Autodesk Inventor part; units mm, degrees
ref_plane "YZ Plane" through (0, 0, 0) normal (1, 0, 0) x (0, 1, 0)
ref_plane "XZ Plane" through (0, 0, 0) normal (0, 1, 0) x (-1, 0, 0)
ref_plane "XY Plane" through (0, 0, 0) normal (0, 0, 1) x (1, 0, 0)
sketch "Sketch1" plane through (0, 0, 0) normal (0, 0, 1) x (1, 0, 0)
  line L0 (0, 0) -> (25.4, 0)
  line L1 (25.4, 0) -> (25.4, -25.4)
  line L2 (25.4, -25.4) -> (0, -25.4)
  line L3 (0, -25.4) -> (0, 0)
  line L4 (1.5875, -23.8125) -> (23.8125, -23.8125)
  line L5 (23.8125, -23.8125) -> (23.8125, -1.5875)
  line L6 (23.8125, -1.5875) -> (1.5875, -1.5875)
  line L7 (1.5875, -1.5875) -> (1.5875, -23.8125)
  dimension "d0" = 25.4
  dimension "d1" = 25.4
  dimension "d2" = 1.5875
extrude "Extrusion1" add sketch "Sketch1" along normal blind 127
sketch "Sketch2" plane through (25.4, -25.4, 0) normal (1, 0, 0) x (0, 0, -1)
  circle A0 centre (-12.7, 12.7) radius 3.3734
  circle A1 centre (-38.1, 12.7) radius 3.3734
  circle A2 centre (-88.9, 12.7) radius 3.3734
  circle A3 centre (-114.3, 12.7) radius 3.3734
  line L0 (0, 25.4) -> (0, 0)
  line L1 (0, 25.4) -> (-127, 25.4)
  line L2 (0, 0) -> (-127, 0)
  line L3 (-127, 0) -> (-127, 25.4)
  dimension "d5" = 6.7469
  dimension "d7" = 12.7
  dimension "d8" = 12.7
  dimension "d9" = 12.7
  dimension "d10" = 38.1
  dimension "d11" = 12.7
  dimension "d12" = 38.1
  dimension "d13" = 12.7
  dimension "d14" = 12.7
extrude "Extrusion2" cut sketch "Sketch2" against normal blind 25.4 contours A0 | A1 | A2 | A3
properties part number "vertical support" material "Aluminum 6061"
Here's how the part is built. I have some questions about the finished solid (model axes, mm). A direction names the side the tool comes from. Give positions to 0.01 mm unless a question says otherwise; leave off trailing zeros. Order: outer loops, then holes, each group sorted by start corner. A loop starts at its lowest first (then second) coordinate and runs counter-clockwise, first axis right, second up. Notation, with made-up numbers: (-3.5, -16) -> (17.5, -16) arc R25 cw to (17.5, 3) -> close; hole circle Ø10 at (-1.5, 56). An arc over 180 degrees is marked (long way). One line per item, written item: value. Start each with the question number.
1. Imagine slicing it at C-C, the plane y = -2.75. List the corners of the cut face in (x, z) for me, plus the area to 3 significant figures.
2. For faces 4 (the face through (13, -1.588, 63)), 5 (the face through (24.617, -13.992, 111.184)), which set-ups out of +Z, -Z, +X, -X, +Y, -Y let a thin tool reach every point of the face, with its end or its side?
3. We'd pull the mould along Y, two halves only. Please class faces 1 (the face through (24.617, -13.992, 34.984)), 2 (the face through (1, -13, 0)), 3 (the face through (13, 0, 63)): released by +Y, released by -Y, zero draft, split by the parting line, or undercut.
4. Imagine slicing it at B-B, the plane z = 88.9. List the corners of the cut face in (x, y) for me.
5. Imagine slicing it at A-A, the plane x = 21.25. List the corners of the cut face in (y, z) for me, plus the area to 3 significant figures.
6. Will this pin go through, and if not, where does the flat tip stop? pin 1 Ø6 at (y, z) = (-12.7, 114.3) entering from +X.
7. Imagine slicing it at D-D, the plane z = 65.5. List the corners of the cut face in (x, y) for me, plus the area to 3 significant figures.
8. I need wall thicknesses on probe 1 along Y at (x, z) = (6.75, 29.5); probe 2 along X at (y, z) = (-6.5, 57); probe 3 along Y at (x, z) = (24.65, 88.9). Which ranges of each line are inside material? Lowest first, please. Write a range as from..to.
Values follow:
1. outline: (0, 0) -> (1.59, 0) -> (1.59, 127) -> (0, 127) -> close; (23.81, 0) -> (25.4, 0) -> (25.4, 127) -> (23.81, 127) -> close
1. area: 403 mm2
2. face 4: +Z, -Z
2. face 5: +X, -X
3. face 1: undercut
3. face 2: zero draft
3. face 3: released by +Y
4. outline: (0, -25.4) -> (25.4, -25.4) -> (25.4, -16.07) -> (23.81, -16.07) -> (23.81, -23.81) -> (1.59, -23.81) -> (1.59, -16.07) -> (0, -16.07) -> close; (0, -9.33) -> (1.59, -9.33) -> (1.59, -1.59) -> (23.81, -1.59) -> (23.81, -9.33) -> (25.4, -9.33) -> (25.4, 0) -> (0, 0) -> close
5. outline: (-25.4, 0) -> (-23.81, 0) -> (-23.81, 127) -> (-25.4, 127) -> close; (-1.59, 0) -> (0, 0) -> (0, 127) -> (-1.59, 127) -> close
5. area: 403 mm2
6. pin 1: passes through
7. outline: (0, -25.4) -> (25.4, -25.4) -> (25.4, 0) -> (0, 0) -> close; hole (1.59, -23.81) -> (23.81, -23.81) -> (23.81, -1.59) -> (1.59, -1.59) -> close
7. area: 151 mm2
8. probe 1: y = -25.4..-23.81, -1.59..0
8. probe 2: x = 0..1.59, 23.81..25.4
8. probe 3: y = -25.4..-16.07, -9.33..0
